Here's how the part is built. I have some questions about the finished solid (model axes, mm). A direction names the side the tool comes from. Coordinates: 2 decimals unless noted, no trailing zeros. Write each loop counter-clockwise with the first axis right and the second up, starting at its lowest first coordinate (ties: lowest second). Pieces come first, ordered by that corner, then holes.
Item 1: We'd pull the mould along X, two halves only. Please class faces 1 (the face through (19, 0, -1)), 2 (the face through (0, 7, -2)), 3 (the face through (11.765, 8.056, -2.218)): +X half, -X half, draft (parallel to the pull), parting line (faces both ways), or undercut.
Item 2: I'm going to push flat-ended pins straight in: pin 1 Ø6 at (x, y) = (11.5, 2.5) entering from +Z; pin 2 Ø4 at (y, z) = (9.5, 2.5) entering from -X; pin 3 Ø1 at (y, z) = (10, 4) entering from +X. Where does each tip first touch, or does it pass through?
Item 3: If we section it at D-D (y = 4.25): Please give me the cut outline in (x, z), then the cut area to 3 significant figures.
Item 4: If we section it at B-B (y = 7.5): Please give me the cut outline in (x, z), then the cut area to 3 significant figures.
Item 5: If I drill on line 1 (Y direction, x = 10, z = -1.85); line 2 (Z direction, x = 4.5, y = 12); line 3 (X direction, y = 2.25, z = 0.5), over which ranges is the centre line in solid material (lowest first)?
Item 6: If we section it at C-C (z = -0.75): Please give me the cut outline in (x, y), then the cut area to 3 significant figures.
Item 7: For faces 4 (the face through (19, 15, -1)), 5 (the face through (12, 7, 0)), which set-ups out of +Z, -Z, +X, -X, +Y, -Y let a thin tool reach every point of the face, with its end or its side?
Item 8: If we section it at A-A (x = 10): Please give me the cut outline in (y, z).
from build123d import *

# Parameters (mm, degrees)
BOSS_EXTRUDE1_DEPTH = 15
SKETCH2_R           = 1.85
CUT_EXTRUDE1_DEPTH  = 37.104189779


with BuildPart() as part:
    # Sketch1 → Boss-Extrude1 (new body)
    with BuildSketch(Plane(origin=(0, 0, 0), x_dir=(1, 0, 0), z_dir=(0, 1, 0))):
        Polygon((20, 4.5), (25, 4.5), (26.048272872, -20), (20, -20), (20, 0), (0, 0), (0, 4.5), align=None)
    extrude(amount=BOSS_EXTRUDE1_DEPTH)

    # Sketch2 → Cut-Extrude1 (cut, through all)
    with BuildSketch(Plane.XY):
        with Locations((10, 7.5)):
            Circle(SKETCH2_R)
    extrude(amount=-CUT_EXTRUDE1_DEPTH, mode=Mode.SUBTRACT)


solid = part.part
Answer list:
1. face 1: draft
1. face 2: -X half
1. face 3: undercut
2. pin 1: stops at z = 0
2. pin 2: stops at x = 20
2. pin 3: stops at x = 25.39
3. outline: (0, -4.5) - (25, -4.5) - (26.05, 20) - (20, 20) - (20, 0) - (0, 0) - close
3. area: 225 mm2
4. outline: (0, -4.5) - (8.15, -4.5) - (8.15, 0) - (0, 0) - close; (11.85, -4.5) - (25, -4.5) - (26.05, 20) - (20, 20) - (20, 0) - (11.85, 0) - close
4. area: 209 mm2
5. line 1: y = 0 to 5.65, 9.35 to 15
5. line 2: z = -4.5 to 0
5. line 3: x = 20 to 25.21
6. outline: (0, 0) - (25.16, 0) - (25.16, 15) - (0, 15) - close; hole circle Ø3.7 at (10, 7.5)
6. area: 367 mm2
7. face 4: +Z, -Z, +X, -X, +Y
7. face 5: +Z, -X, +Y, -Y
8. outline: (0, -4.5) - (5.65, -4.5) - (5.65, 0) - (0, 0) - close; (9.35, -4.5) - (15, -4.5) - (15, 0) - (9.35, 0) - close
